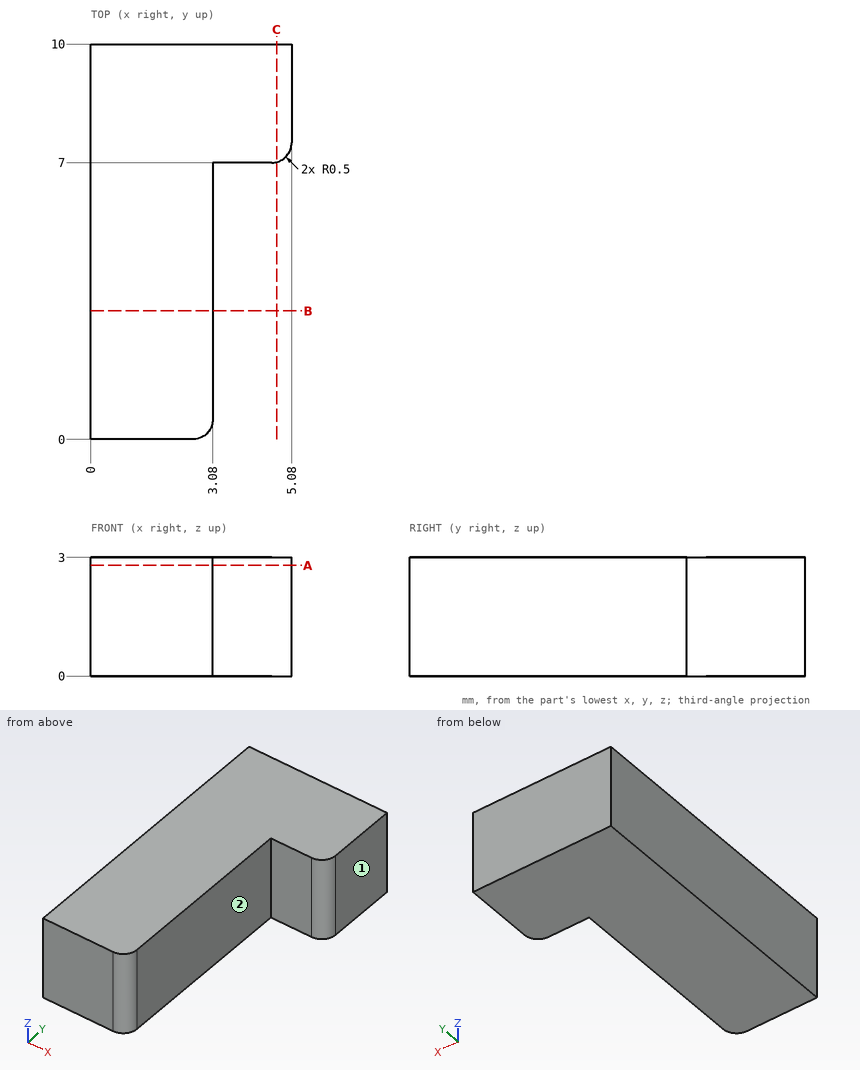
Answer from the drawing. Dimensions are ordinates in mm from the lowest x, y and z of the part. A direction names the side the tool comes from. Give positions to 0.01 mm unless a question says otherwise; leave off trailing zeros. Loops run counter-clockwise (first coordinate to the right, second up) from the corner with the lowest first, then second, coordinate; pieces in that order, holes last.
Item 1: A cutting plane is placed at A-A (z = 2.8). Give the vertices of the cut face in (x, y), then the cut area to 3 significant figures.
Derived:
outline: (0, 0) - (2.58, 0) arc R0.5 ccw to (3.08, 0.5) - (3.08, 7) - (4.58, 7) arc R0.5 ccw to (5.08, 7.5) - (5.08, 10) - (0, 10) - close
area: 36.7 mm2
Item 2: A tool of negligible diameter and unlimited length cuts with its end or side. For the marked faces 1 and 2, from which of +Z, -Z, +X, -X, +Y, -Y can it reach the whole face along a straight path? Write none if from no direction.
Derived:
face 1: +Z, -Z, +X, +Y, -Y
face 2: +Z, -Z, +X, -Y
Item 3: Each of these flat-tipped pins is pushed along its axis until it touches: pin 1 Ø3 at (x, y) = (3.5, 5.5) entering from -Z; pin 2 Ø0.8 at (x, z) = (4, 1) entering from -Y; pin 3 Ø1 at (x, y) = (4.5, 2) entering from -Z. Where does it stop, or does it pass through?
Derived:
pin 1: stops at z = 0
pin 2: stops at y = 7
pin 3: passes through
Item 4: A cutting plane is placed at C-C (x = 4.7). Give the vertices of the cut face in (y, z), then the cut area to 3 significant figures.
Derived:
outline: (7.01, 0) - (10, 0) - (10, 3) - (7.01, 3) - close
area: 8.96 mm2
Item 5: A cutting plane is placed at B-B (y = 3.25). Give the vertices of the cut face in (x, z), then the cut area to 3 significant figures.
Derived:
outline: (0, 0) - (3.08, 0) - (3.08, 3) - (0, 3) - close
area: 9.24 mm2
Item 6: Find the intervals of material crossed by line 1 along Y through (x, z) = (4.5, 2.05); line 2 along X through (y, z) = (5.75, 0.85); line 3 along Y through (x, z) = (2.75, 2.6), in increasing order.
Derived:
line 1: y = 7 to 10
line 2: x = 0 to 3.08
line 3: y = 0.03 to 10
